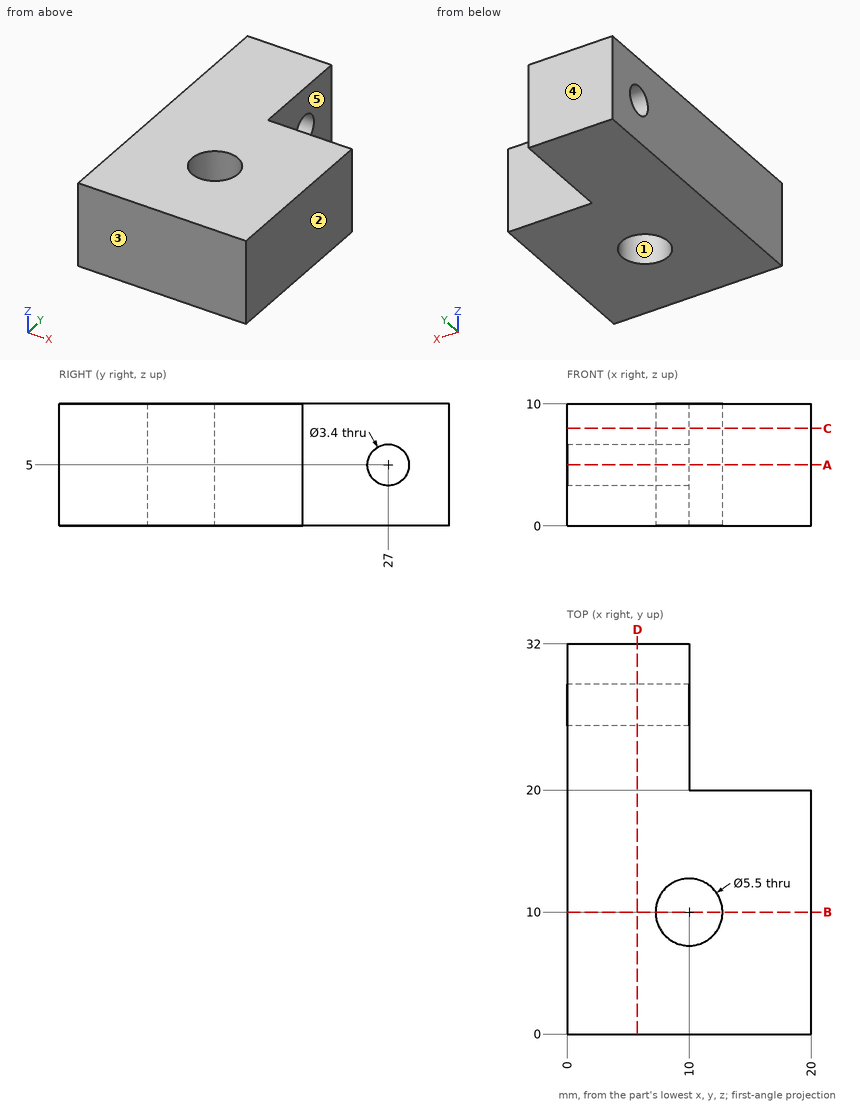
Could you check a few things on this drawing? It's one solid part, dimensions in mm from its lowest x, y, z. A direction names the side the tool comes from. Give positions to 0.01 mm unless a question says otherwise; leave off trailing zeros. Loops run counter-clockwise (first coordinate to the right, second up) from the corner with the lowest first, then second, coordinate; pieces in that order, holes last. Notation, with made-up numbers: (33, -36.75) -> (62, -36.75) arc R17 cw to (62, -25.75) -> close; hole circle Ø5 at (-29.75, -12.75). An arc over 180 degrees is marked (long way). Use one line per item in the form item = value. Start each with the question number.
1) For P1, Ø1.5, axis at x = 11, z = 7.5, coming from the +Y side; P2, Ø5, axis at y = 27, z = 5, coming from the +X side, each with a flat end and sliding along its axis, tell me the tip position at first contact or that it passes through.
2) Imagine slicing it at C-C (z = 8). Please give me the cut outline in (x, y).
3) Thinking about a two-plate mould opening in X: for the marked faces 1, 2 and 3, which applies, +X half, -X half, draft (parallel to the pull), parting line (faces both ways), or undercut?
4) Imagine slicing it at B-B (y = 10). Please give me the cut outline in (x, z), then the cut area to 3 significant figures.
5) Please list where these lines run through material, in increasing order: line 1 along Y through (x, z) = (8, 5); line 2 along Y through (x, z) = (2, 5); line 3 along X through (y, z) = (21, 4.75).
6) Imagine slicing it at D-D (x = 5.75). Please give me the cut outline in (y, z).
7) Imagine slicing it at A-A (z = 5). Please give me the cut outline in (x, y).
8) Which directions (+Z, -Z, +X, -X, +Y, -Y) give clear straight access to the entire face, cutting with the end or side of a thin tool? Please do the marked faces 4 and 5.
Check values:
q1.P1 = 20
q1.P2 = 10
q2.outline = (0, 0) -> (20, 0) -> (20, 20) -> (10, 20) -> (10, 32) -> (0, 32) -> close; hole circle Ø5.5 at (10, 10)
q3.face_1 = undercut
q3.face_2 = +X half
q3.face_3 = draft
q4.outline = (0, 0) -> (7.25, 0) -> (7.25, 10) -> (0, 10) -> close; (12.75, 0) -> (20, 0) -> (20, 10) -> (12.75, 10) -> close
q4.area = 145 mm^2
q5.line_1 = 0 to 8.11, 11.89 to 25.3, 28.7 to 32
q5.line_2 = 0 to 25.3, 28.7 to 32
q5.line_3 = 0 to 10
q6.outline = (0, 0) -> (32, 0) -> (32, 10) -> (0, 10) -> close; hole circle Ø3.4 at (27, 5)
q7.outline = (0, 0) -> (20, 0) -> (20, 20) -> (10, 20) -> (10, 25.3) -> (0, 25.3) -> close; (0, 28.7) -> (10, 28.7) -> (10, 32) -> (0, 32) -> close; hole circle Ø5.5 at (10, 10)
q8.face_4 = +Z, -Z, +X, -X, +Y
q8.face_5 = +Z, -Z, +X, +Y
